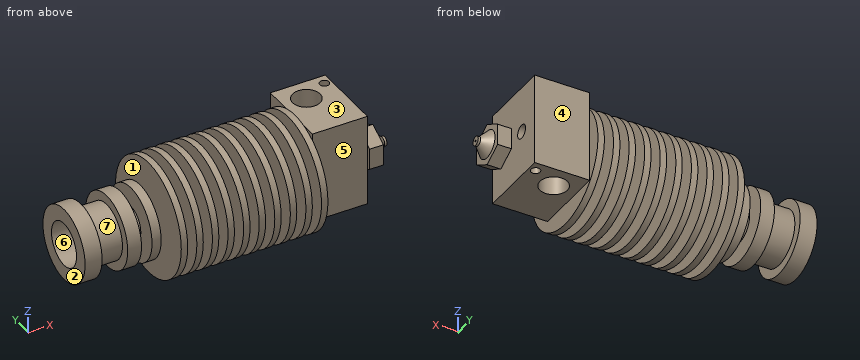
```python
from build123d import *

# Parameters (mm, degrees)
BOSS_EXTRUDE1_DEPTH = 3
BOSS_EXTRUDE2_START = -10
SKETCH3_W           = 12
SKETCH3_H           = 16
SKETCH3_R           = 3
SKETCH3_R_2         = 1
BOSS_EXTRUDE2_DEPTH = 20
SKETCH4_R           = 1.5
CUT_EXTRUDE5_DEPTH  = 12
CUT_EXTRUDE6_START  = -13.5
SKETCH5_R           = 1
CUT_EXTRUDE6_DEPTH  = 18.2


with BuildPart() as part:
    # Sketch1 → Revolve1 (revolve)
    with BuildSketch(Plane.XY, mode=Mode.PRIVATE) as revolve1_sk:
        Polygon((0, 8), (3.7, 8), (3.7, 6), (9.3, 6), (9.3, 8), (12.3, 8), (12.3, 3.75), (14.6, 3.75), (14.6, 8), (16.6, 8), (16.6, 3.75), (18.4, 3.75), (18.4, 12.5), (19.8, 12.5), (19.8, 3.75), (21.8, 3.75), (21.8, 12.5), (23.2, 12.5), (23.2, 3.75), (25.2, 3.75), (25.2, 12.5), (26.6, 12.5), (26.6, 3.75), (28.6, 3.75), (28.6, 12.5), (30, 12.5), (30, 3.75), (32, 3.75), (32, 12.5), (33.4, 12.5), (33.4, 3.75), (35.4, 3.75), (35.4, 12.5), (36.8, 12.5), (36.8, 3.75), (38.8, 3.75), (38.8, 12.5), (40.2, 12.5), (40.2, 3.75), (42.2, 3.75), (42.2, 12.5), (43.6, 12.5), (43.6, 3.75), (45.6, 3.75), (45.6, 12.5), (47, 12.5), (47, 3.75), (49, 3.75), (49, 12.5), (50.4, 12.5), (50.4, 3), (64.4, 3), (64.4, 4), (67.4, 4), (67.4, 3), (69.4, 1), (69.9, 1), (69.9, 0.2), (69.4, 0.2), (68.6, 1), (11.75, 1), (8, 4.75), (0, 4.75), align=None)
    revolve(revolve1_sk.sketch.rotate(Axis((0, 0, 0), (1, 0, 0)), 180), axis=Axis((0, 0, 0), (1, 0, 0)))

    # Sketch2 → Boss-Extrude1 (add)
    with BuildSketch(Plane.ZY.offset(-64.4)):
        Polygon((2.309401077, 4), (-2.309401077, 4), (-4.618802154, 0), (-2.309401077, -4), (2.309401077, -4), (4.618802154, 0), align=None)
    extrude(amount=-BOSS_EXTRUDE1_DEPTH)

    # Sketch3 → Boss-Extrude2 (add)
    with BuildSketch(Plane.XY.offset(BOSS_EXTRUDE2_START)):
        with Locations((57.9, 4)):
            Rectangle(SKETCH3_W, SKETCH3_H)
        with Locations((56.9, 7)):
            Circle(SKETCH3_R, mode=Mode.SUBTRACT)
        with Locations((62.4, 9.7)):
            Circle(SKETCH3_R_2, mode=Mode.SUBTRACT)
    extrude(amount=BOSS_EXTRUDE2_DEPTH)

    # Sketch4 → Cut-Extrude5 (cut)
    with BuildSketch(Plane(origin=(63.9, 0, 0), x_dir=(0, 0, -1), z_dir=(1, 0, 0))):
        with Locations((0, 7)):
            Circle(SKETCH4_R)
    extrude(amount=-CUT_EXTRUDE5_DEPTH, mode=Mode.SUBTRACT)

    # Sketch5 → Cut-Extrude6 (cut)
    with BuildSketch(Plane(origin=(63.9, 0, 0), x_dir=(0, 0, -1), z_dir=(1, 0, 0)).offset(CUT_EXTRUDE6_START)):
        with Locations(Location((0, 0, 0), (0, 0, 270))):
            Circle(SKETCH5_R)
    extrude(amount=CUT_EXTRUDE6_DEPTH, mode=Mode.SUBTRACT)


solid = part.part
```
Geometry check sheet. Reference: the model listing, model coordinates, mm. Face numbers are marked on the shaded views. A direction names the side the tool comes from. Give positions to 0.01 mm unless a question says otherwise; leave off trailing zeros. Loops run counter-clockwise (first coordinate to the right, second up) from the corner with the lowest first, then second, coordinate; pieces in that order, holes last. Notation, with made-up numbers: M -7.75,13 L 20.25,13 A29 cw 20.25,50 Z; hole C 55.25,49 d9. An arc over 180 degrees is marked long. Write item = value, one per line. Start each with the question number.
1. Draft check along X on the marked faces 1, 2 and 3. Enter one of: +X half, -X half, draft (parallel to the pull), parting line (faces both ways), or undercut.
2. Tool access check on the marked faces 4, 5, 6 and 7. Record the directions out of +Z, -Z, +X, -X, +Y, -Y that give a thin tool (end or side, any length) a straight path to the whole face; none if there is none.
3. Thickness scan on probe 1 along Z at (x, y) = (69.8, 0); probe 2 along X at (y, z) = (-3, -0.5); probe 3 along X at (y, z) = (11, -6.75). Record the ranges inside material, lowest first.
4. Section check B-B, the plane z = -6.75. Give the number of separate pieces and of enclosed holes in the cut face, plus the area to 3 significant figures.
5. Section check A-A, the plane x = 62.4. Enter the section's corners in (y, z), plus the area to 3 significant figures.
6. Go/stop test with flat-tipped pins: P1, Ø4, axis at x = 44, z = 7, coming from the +Y side; P2, Ø5, axis at x = 29, y = 7.5, coming from the -Z side; P3, Ø8, axis at y = -4, z = 7.5, coming from the +X side. Record where each tip stops, or that it passes through.
Values follow:
q1.face_1 = undercut
q1.face_2 = -X half
q1.face_3 = draft
q2.face_4 = +Z, -Z, +X, +Y
q2.face_5 = +Z, -Z, +X, -Y
q2.face_6 = -X
q2.face_7 = none
q3.probe_1 = -1 to -0.2, 0.2 to 1
q3.probe_2 = 9.71 to 50.4, 51.9 to 63.9, 64.4 to 67.4
q3.probe_3 = 51.9 to 63.9
q4.separate_pieces = 14
q4.enclosed_holes = 2
q4.area = 530 mm^2
q5.outline = M -4,-10 L 8.7,-10 L 8.7,10 L -4,10 Z; M 10.7,-10 L 12,-10 L 12,10 L 10.7,10 Z; hole C 0,0 d2; hole C 7,0 d3
q5.area = 270 mm^2
q6.P1 = 11.44
q6.P2 = -11.46
q6.P3 = 63.9
